```python
from build123d import *

# Parameters (mm, degrees)
SKETCH1_W           = 30
SKETCH1_H           = 41
BOSS_EXTRUDE1_DEPTH = 105
SKETCH2_W           = 21.801991159
SKETCH2_H           = 5.700874013
SKETCH2_W_2         = 22.379782444
SKETCH2_H_2         = 5.277160404
BOSS_EXTRUDE2_DEPTH = 5


with BuildPart() as part:
    # Sketch1 → Boss-Extrude1 (new body)
    with BuildSketch(Plane(origin=(0, 0, 0), x_dir=(1, 0, 0), z_dir=(0, 1, 0))):
        Rectangle(SKETCH1_W, SKETCH1_H)
    extrude(amount=BOSS_EXTRUDE1_DEPTH)

    # Sketch2 → Boss-Extrude2 (add)
    with BuildSketch(Plane.XZ):
        with Locations((-0.134817966, 15.234430217)):
            Rectangle(SKETCH2_W, SKETCH2_H)
        with Locations((0.462233028, -15.061092832)):
            Rectangle(SKETCH2_W_2, SKETCH2_H_2)
    extrude(amount=BOSS_EXTRUDE2_DEPTH)


solid = part.part
```
The model under review builds one solid part; all positions refer to its coordinate system, in mm. A direction names the side the tool comes from. Round coordinates to 2 decimals unless told otherwise and drop trailing zeros. Order: outer loops, then holes, each group sorted by start corner. A loop starts at its lowest first (then second) coordinate and runs counter-clockwise, first axis right, second up. Notation, with made-up numbers: (-2, 63.5) -> (2, 63.5) arc R11 ccw to (2, 67.5) -> close; hole circle Ø5 at (-6, 57). An arc over 180 degrees is marked (long way). Use a Markdown table: item, result.
Q1. For line 1 (Y direction, x = 7.25, z = -11), list the stretches that pass through material, from the lowest coordinate up.
Values:
| item | result |
|---|---|
| line 1 | y = 0 to 105 |
Q2. Tool access review of faces 1 (the flat face through (11.652, -2, -15)), 2 (the flat face through (0, -2, 18.085)), 3 (the flat face through (0, -2, -12.423)), 4 (the flat face through (-10.728, -2, -15)): name each direction out of +Z, -Z, +X, -X, +Y, -Y from which nothing blocks a thin tool from reaching the whole face with its end or side.
Values:
| item | result |
|---|---|
| face 1 | +Z, -Z, +X, -Y |
| face 2 | +Z, +X, -X, -Y |
| face 3 | +X, -X, -Y |
| face 4 | -Z, -X, -Y |
Q3. We need section A-A on x = -9.5. Write out the cut boundary in (y, z).
Values:
| item | result |
|---|---|
| outline | (-5, -17.7) -> (0, -17.7) -> (0, -20.5) -> (105, -20.5) -> (105, 20.5) -> (0, 20.5) -> (0, 18.08) -> (-5, 18.08) -> (-5, 12.38) -> (0, 12.38) -> (0, -12.42) -> (-5, -12.42) -> close |
Q4. We need section B-B on z = -6.5. Write out the cut boundary in (x, y), then the cut area to 3 significant figures.
Values:
| item | result |
|---|---|
| outline | (-15, 0) -> (15, 0) -> (15, 105) -> (-15, 105) -> close |
| area | 3,150 mm^2 |
Q5. Clearance check with flat-ended pins moving along their axes: P1, Ø15, axis at x = 2, z = -4.5, coming from the -Y side; P2, Ø1.5, axis at x = -0.5, y = -1.5, coming from the +Z side; P3, Ø1.5, axis at y = -3.5, z = 14, coming from the -X side. State where each tip first meets the part, or that it passes through.
Values:
| item | result |
|---|---|
| P1 | stops at y = 0 |
| P2 | stops at z = 18.08 |
| P3 | stops at x = -11.04 |
